Work out the finished part from the listing and answer in its coordinate system (mm). Face numbers are marked on the shaded views. A direction names the side the tool comes from. Round coordinates to 2 decimals unless told otherwise and drop trailing zeros. Write each loop counter-clockwise with the first axis right and the second up, starting at its lowest first coordinate (ties: lowest second). Pieces come first, ordered by that corner, then holes. Notation, with made-up numbers: (-11, 35) - (7, 35) arc R19 ccw to (7, 44) - close; hole circle Ø7 at (81.25, 31.5). An arc over 180 degrees is marked (long way). Answer as a JSON object with one key per item and string values.
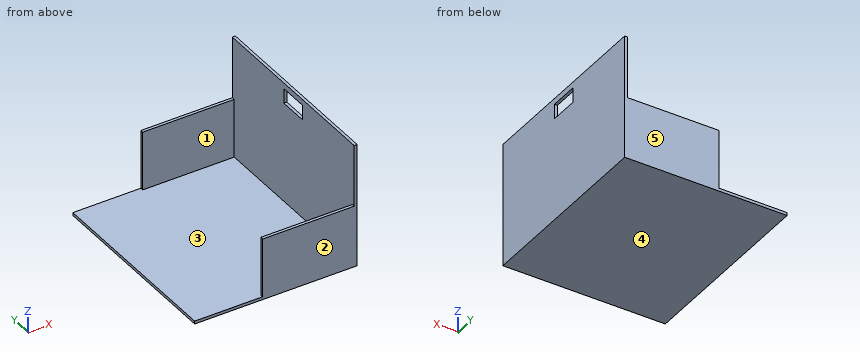
Autodesk Inventor part; units mm, degrees
ref_plane "Work Plane2" through (21.7343, 0, 1) normal (0, -1, 0) x (1, 0, 0)
ref_plane "YZ Plane" through (0, 0, 0) normal (1, 0, 0) x (0, 1, 0)
ref_plane "XZ Plane" through (0, 0, 0) normal (0, 1, 0) x (-1, 0, 0)
sketch "Sketch2" plane through (0, 0, 0) normal (0, 0, 1) x (1, 0, 0)
  line L0 (-32.2657, 32.5) -> (21.7343, 32.5)
  line L1 (21.7343, 32.5) -> (21.7343, -32.5)
  line L2 (21.7343, -32.5) -> (-32.2657, -32.5)
  line L3 (-32.2657, -32.5) -> (-32.2657, 32.5)
  line L4 (-43.0657, 0) -> (32.5343, 0)
  point P0 (0, 0)
  dimension "d13" = 54
  dimension "d14" = 65
extrude "Extrusion2" add sketch "Sketch2" along normal blind 1
sketch "Sketch3" plane through (21.7343, -32.5, 0) normal (1, 0, 0) x (0, 0, -1)
  line L0 (0, 0) -> (-21, 0)
  line L1 (-21, 0) -> (-21, 65)
  line L2 (-21, 65) -> (0, 65)
  line L3 (0, 65) -> (0, 0)
  line L4 (-1, 0) -> (-1, 65)
  line L5 (0, 65) -> (0, 0)
  line L6 (0, 65) -> (-1, 65)
  point P0 (0, 32.5)
  dimension "d9" = 20
extrude "Extrusion3" add sketch "Sketch3" along normal blind 1
sketch "Sketch4" plane through (21.7343, 32.5, 21) normal (0, 1, 0) x (1, 0, 0)
  line L0 (0, 20) -> (-54, 20)
  line L1 (0, 0) -> (0, 20)
  line L2 (-31, 20) -> (0, 20)
  line L3 (0, 20) -> (0, 0)
  line L4 (0, 0) -> (-31, 0)
  line L5 (-31, 0) -> (-31, 20)
  line L6 (1, 21) -> (1, 0)
  point P0 (-21.7343, 21)
  dimension "d15" = 32
extrude "Extrusion4" add sketch "Sketch4" against normal blind 1
ref_plane "Work Plane2" through (21.7343, 0, 1) normal (0, -1, 0) x (1, 0, 0)
mirror "Mirror3" about plane through (21.7343, 0, 1) normal (0, -1, 0) of "Extrusion4"
sketch "Sketch5" plane through (22.7343, -32.5, 21) normal (0, 0, 1) x (1, 0, 0)
  line L0 (-1, 64) -> (-32, 64)
  line L1 (-1, 64) -> (-1, 65)
  line L2 (-55, 65) -> (0, 65)
  line L3 (-32, 1) -> (-1, 1)
  line L4 (-1, 1) -> (-1, 0)
  line L5 (0, 0) -> (-55, 0)
  line L6 (-1, 1) -> (-1, 64)
  line L7 (0, 65) -> (0, 0)
  line L8 (0, 65) -> (-32, 65)
  line L9 (0, 0) -> (-32, 0)
  point P0 (-22.7343, 32.5)
extrude "Extrusion5" add sketch "Sketch5" along normal blind 21
sketch "Sketch6" plane through (22.7343, -32.5, 0) normal (1, 0, 0) x (0, 0, -1)
  line L0 (-35, 37.5) -> (-40, 37.5)
  line L1 (-40, 37.5) -> (-40, 27.5)
  line L2 (-40, 27.5) -> (-35, 27.5)
  line L3 (-35, 27.5) -> (-35, 37.5)
  line L4 (-42, 0) -> (-42, 65)
  line L5 (0, 32.5) -> (-42, 32.5) construction
  dimension "d18" = 2
  dimension "d19" = 5
  dimension "d20" = 10
extrude "Extrusion6" cut sketch "Sketch6" against normal up to next
properties part number "ProjectXBaseTop"
Item 1: Consider line 1 along Y through (x, z) = (1.5, 18); line 2 along X through (y, z) = (-4.5, 6.5); line 3 along Z through (x, y) = (-19.5, 28.5). Determine where each line is inside the solid, lowest interval first.
Results found:
{"line 1": "-32.5 to -31.5, 31.5 to 32.5", "line 2": "21.73 to 22.73", "line 3": "0 to 1"}
Item 2: Each of these flat-tipped pins is pushed along its axis until it touches: P1, Ø1.5, axis at x = 11.5, y = -7.5, coming from the +Z side; P2, Ø0.5, axis at y = -32, z = 6.5, coming from the -X side; P3, Ø1.5, axis at x = -10.5, z = 18.5, coming from the +Y side; P4, Ø12.5, axis at y = -5, z = 17, coming from the -X side. Where does it stop, or does it pass through?
Results found:
{"P1": "z = 1", "P2": "x = -9.27", "P3": "through", "P4": "x = 21.73"}
Item 3: A cutting plane is placed at C-C (x = -2). Write down the section's boundary in (y, z), and give its area (3 significant figures).
Results found:
{"outline": "(-32.5, 0) - (32.5, 0) - (32.5, 21) - (31.5, 21) - (31.5, 1) - (-31.5, 1) - (-31.5, 21) - (-32.5, 21) - close", "area": "105 mm²"}
Item 4: A cutting plane is placed at A-A (z = 14.5). Write down the section's boundary in (x, y).
Results found:
{"outline": "(-9.27, -32.5) - (22.73, -32.5) - (22.73, 32.5) - (-9.27, 32.5) - (-9.27, 31.5) - (21.73, 31.5) - (21.73, -31.5) - (-9.27, -31.5) - close"}
Item 5: A cutting plane is placed at D-D (x = -18). Write down the section's boundary in (y, z).
Results found:
{"outline": "(-32.5, 0) - (32.5, 0) - (32.5, 1) - (-32.5, 1) - close"}
Item 6: A cutting plane is placed at B-B (y = 10.5). Write down the section's boundary in (x, z), and give its area (3 significant figures).
Results found:
{"outline": "(-32.27, 0) - (22.73, 0) - (22.73, 42) - (21.73, 42) - (21.73, 1) - (-32.27, 1) - close", "area": "96.0 mm²"}
Item 7: For the marked faces 1 and 2, determine the directions among +Z, -Z, +X, -X, +Y, -Y from which every point of the face is accessible in a straight line to the end or side of a thin tool.
Results found:
{"face 1": "+Z, -X", "face 2": "+Z, -Z, +X, -X, -Y"}
Item 8: Determine the mould class of the marked faces 3, 4 and 5 for opening direction Y: pulls with the +Y half, pulls with the -Y half, needs draft (parallel to the pull), parting line crosses it, or undercut.
Results found:
{"face 3": "undercut", "face 4": "needs draft", "face 5": "pulls with the +Y half"}
